Could you check a few things on this model? Use its own coordinates, in mm. A direction names the side the tool comes from. Round coordinates to 2 decimals unless told otherwise and drop trailing zeros. Loops run counter-clockwise (first coordinate to the right, second up) from the corner with the lowest first, then second, coordinate; pieces in that order, holes last. Notation, with made-up numbers: (40.5, 5.25) -> (93.5, 5.25) arc R20 cw to (93.5, 32.25) -> close; hole circle Ø5 at (21, 35.5). An arc over 180 degrees is marked (long way). Use CSV: the item, a comma, the result in double quotes. Start each with the question number.
```python
from build123d import *

# Parameters (mm, degrees)
SKETCH_W     = 15
SKETCH_H     = 15
PAD_DEPTH    = 15
SKETCH001_W  = 12
SKETCH001_H  = 12
PAD001_DEPTH = 40
SKETCH003_W  = 12
SKETCH003_H  = 12
PAD003_DEPTH = 40
SKETCH002_W  = 12
SKETCH002_H  = 12
PAD002_DEPTH = 40
SKETCH004_W  = 12
SKETCH004_H  = 12
PAD004_DEPTH = 40


with BuildPart() as pad001:
    # Sketch → Pad (new body)
    with BuildSketch(Plane.XY):
        Rectangle(SKETCH_W, SKETCH_H)
    extrude(amount=PAD_DEPTH)

    # Sketch001 → Pad001 (new body)
    with BuildSketch(Plane.XY.offset(15)):
        Rectangle(SKETCH001_W, SKETCH001_H)
    extrude(amount=PAD001_DEPTH)


with BuildPart() as pad003:
    # Pad003 base: copy of Pad001
    add(pad001.part)

    # Sketch003 → Pad003 (new body)
    with BuildSketch(Plane(origin=(0, 0, 0), x_dir=(1, 0, 0), z_dir=(0, 0, -1))):
        Rectangle(SKETCH003_W, SKETCH003_H)
    extrude(amount=PAD003_DEPTH)


with BuildPart() as fusion:
    # Pad002 base: copy of Pad001
    add(pad001.part)

    # Sketch002 → Pad002 (new body)
    with BuildSketch(Plane(origin=(0, 7.5, 0), x_dir=(-1, 0, 0), z_dir=(0, 1, 0))):
        with Locations((0, 7.5)):
            Rectangle(SKETCH002_W, SKETCH002_H)
    extrude(amount=PAD002_DEPTH)

    # Sketch004 → Pad004 (new body)
    with BuildSketch(Plane.YZ.offset(7.5)):
        with Locations((0, 7.5)):
            Rectangle(SKETCH004_W, SKETCH004_H)
    extrude(amount=PAD004_DEPTH)

    # Fusion: union Pad003
    add(pad003.part)


solid = fusion.part
```
1. Suppose I cut it at A-A (y = 0.5). List the corners of the cut face in (x, z) for me, then the cut area to 4 significant figures.
2. For faces 1 (the face through (27, 0, 1.5)), 2 (the face through (0, 27, 1.5)), 3 (the face through (0, 27, 13.5)), 4 (the face through (6, 0, 35)), which set-ups out of +Z, -Z, +X, -X, +Y, -Y let a thin tool reach every point of the face, with its end or its side?
3. If I drill on L1, parallel to Y at x = 3, z = 51; L2, parallel to Z at x = 4, y = 13, over which ranges is the centre line in solid material (lowest first)?
4. Will these pins go through, and if not, where does the flat tip stop? pin 1 (6 mm diameter, centred on x = -3, y = 36, fed in from +Z); pin 2 (6 mm diameter, centred on x = 21.5, y = 1.5, fed in from -Z); pin 3 (13 mm diameter, centred on x = -3, z = -22, fed in from +Y).
5. Suppose I cut it at D-D (y = 23.5). List the corners of the cut face in (x, z) for me.
6. Suppose I cut it at C-C (z = -4.5). List the corners of the cut face in (x, y) for me.
Geometry check:
1,outline,"(-7.5, 0) -> (-6, 0) -> (-6, -40) -> (6, -40) -> (6, 0) -> (7.5, 0) -> (7.5, 1.5) -> (47.5, 1.5) -> (47.5, 13.5) -> (7.5, 13.5) -> (7.5, 15) -> (6, 15) -> (6, 55) -> (-6, 55) -> (-6, 15) -> (-7.5, 15) -> close"
1,area,"1,665 mm²"
2,face 1,"-Z, +X, +Y, -Y"
2,face 2,"-Z, +X, -X, +Y"
2,face 3,"+Z, +X, -X, +Y"
2,face 4,"+Z, +X, +Y, -Y"
3,L1,"y = -6 to 6"
3,L2,"z = 1.5 to 13.5"
4,pin 1,"stops at z = 13.5"
4,pin 2,"stops at z = 1.5"
4,pin 3,"stops at y = 6"
5,outline,"(-6, 1.5) -> (6, 1.5) -> (6, 13.5) -> (-6, 13.5) -> close"
6,outline,"(-6, -6) -> (6, -6) -> (6, 6) -> (-6, 6) -> close"
